Job drawing, mm, ordinate dimensions from the low corner. One solid piece. A direction names the side the tool comes from. Give positions to 0.01 mm unless a question says otherwise; leave off trailing zeros. Loops run counter-clockwise (first coordinate to the right, second up) from the corner with the lowest first, then second, coordinate; pieces in that order, holes last. Notation, with made-up numbers: M 65.5,66.25 L 72.5,66.25 A20 cw 72.5,85.25 Z; hole C 42.25,20.25 d3. An arc over 180 degrees is marked long. One line per question, with ' | ' between items.
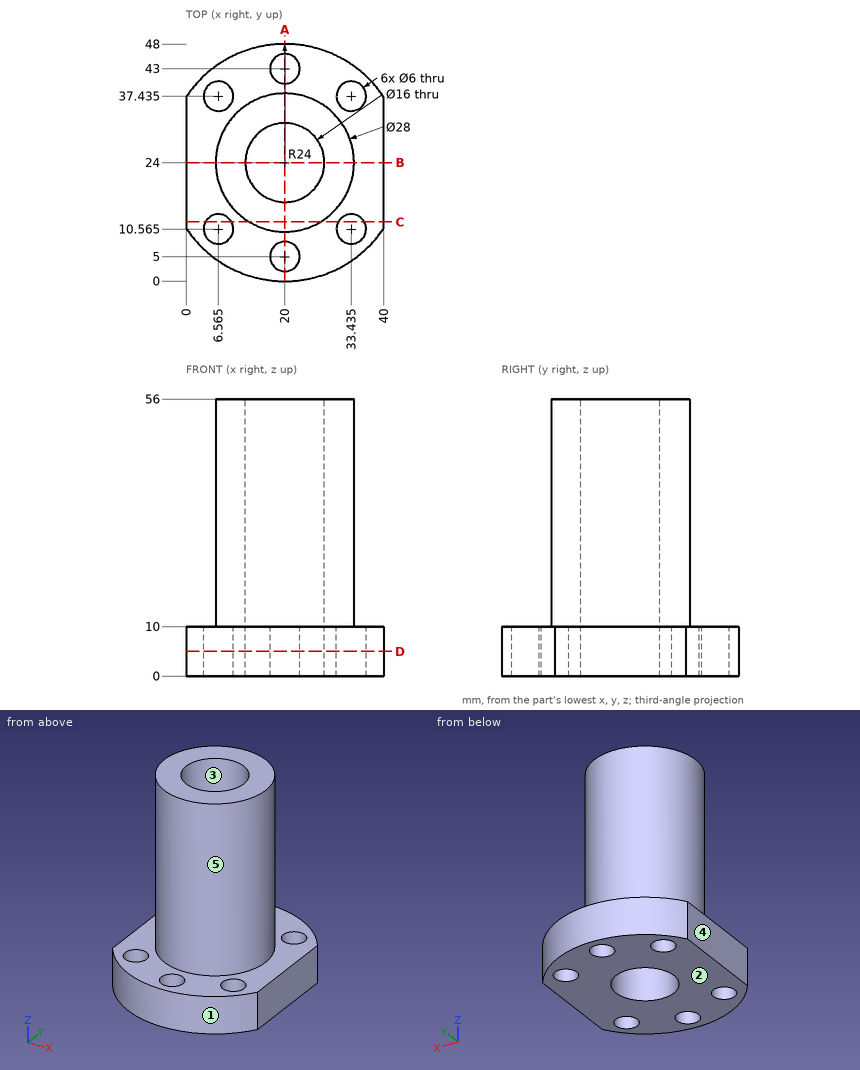
Item 1: Saw through at C-C on y = 12. Give the cut face in (x, z).
Conclusion:
outline: M 0,0 L 3.93,0 L 3.93,10 L 0,10 Z; M 9.2,0 L 30.8,0 L 30.8,10 L 27.21,10 L 27.21,56 L 12.79,56 L 12.79,10 L 9.2,10 Z; M 36.07,0 L 40,0 L 40,10 L 36.07,10 Z
Item 2: Drill centre lines: line 1 along Y through (x, z) = (20, 41.5); line 2 along X through (y, z) = (12.5, 53); line 3 along Z through (x, y) = (12, 45). Where is each one in solid material? Low to high. Write a range as [from, to].
Conclusion:
line 1: [10, 16], [32, 38] | line 2: [12.02, 27.98] | line 3: [0, 10]
Item 3: 3-axis set-ups, long thin cutter, end or side, ignore diameter. For the marked faces 4 and 5: which of +Z, -Z, +X, -X, +Y, -Y reach the whole face in a straight line?
Conclusion:
face 4: +Z, -Z, -X, +Y, -Y | face 5: +Z
Item 4: Mould opens along X. For the marked faces 1, 2 and 3 say: pulls with the +X half, pulls with the -X half, needs draft (parallel to the pull), parting line crosses it, or undercut.
Conclusion:
face 1: parting line crosses it | face 2: needs draft | face 3: undercut
Item 5: Saw through at B-B on y = 24. Give the cut face in (x, z).
Conclusion:
outline: M 0,0 L 12,0 L 12,56 L 6,56 L 6,10 L 0,10 Z; M 28,0 L 40,0 L 40,10 L 34,10 L 34,56 L 28,56 Z
Item 6: Drop flat-ended pins along their axis: P1, Ø8, axis at x = 6.56, y = 37.44, coming from the +Z side; P2, Ø4, axis at x = 15, z = 41, coming from the +Y side; P3, Ø5.5, axis at x = 20, y = 5, coming from the +Z side; P4, Ø10, axis at x = 21, z = 30, coming from the -Y side. Give the stop position or say it passes through.
Conclusion:
P1: z = 10 | P2: y = 37.67 | P3: through | P4: y = 10
Item 7: Saw through at A-A on x = 20. Give the cut face in (y, z).
Conclusion:
outline: M 0,0 L 2,0 L 2,10 L 0,10 Z; M 8,0 L 16,0 L 16,56 L 10,56 L 10,10 L 8,10 Z; M 32,0 L 40,0 L 40,10 L 38,10 L 38,56 L 32,56 Z; M 46,0 L 48,0 L 48,10 L 46,10 Z
Item 8: Saw through at D-D on z = 5. Give the cut face in (x, y) (1 decimal).
Conclusion:
outline: M 0,10.7 A24 ccw 40,10.7 L 40,37.3 A24 ccw 0,37.3 Z; hole C 6.6,10.6 d6; hole C 6.6,37.4 d6; hole C 20,24 d16; hole C 20,5 d6; hole C 20,43 d6; hole C 33.4,10.6 d6; hole C 33.4,37.4 d6
